from build123d import *

# Parameters (mm, degrees)
BOSS_EXTRUDE1_DEPTH     = 3
FILLET1_R               = 5
CUT_EXTRUDE1_DEPTH      = 165.496200564
CUT_EXTRUDE1_DEPTH_BACK = 165.496200564
SKETCH2_R               = 1.5
CUT_EXTRUDE2_DEPTH      = 165.496200694
CUT_EXTRUDE2_DEPTH_BACK = 165.496200694
SKETCH3_R               = 2.5
CUT_EXTRUDE3_DEPTH      = 165.496200694
CUT_EXTRUDE3_DEPTH_BACK = 165.496200694
SKETCH4_R               = 3.75
SKETCH4_R_2             = 2.75
SKETCH4_W               = 71.5
SKETCH4_H               = 25
SKETCH5_R               = 1.5
BOSS_EXTRUDE2_DEPTH     = 25


with BuildPart() as part:
    # Sketch1 → Boss-Extrude1 (new body)
    with BuildSketch(Plane(origin=(0, 0, 0), x_dir=(1, 0, 0), z_dir=(0, 1, 0))):
        with BuildLine():
            Line((0, 5), (150, 5))
            ThreePointArc((150, 5), (153.535533906, 3.535533906), (155, 0))
            Line((155, 0), (155, -50))
            ThreePointArc((155, -50), (153.535533906, -53.535533906), (150, -55))
            Line((150, -55), (0, -55))
            ThreePointArc((0, -55), (-3.535533906, -53.535533906), (-5, -50))
            Line((-5, -50), (-5, 0))
            ThreePointArc((-5, 0), (-3.535533906, 3.535533906), (0, 5))
        make_face()
    extrude(amount=BOSS_EXTRUDE1_DEPTH)

    # Fillet1
    # the kernel refuses this fillet: 5 mm, written as the material it takes off along each edge
    with BuildSketch(Plane(origin=(0, 3, 50), x_dir=(0, 0, 1), z_dir=(1, 0, 0))) as fillet1_piece_1:
        with BuildLine():
            CenterArc((0.417424305, 5), FILLET1_R, 270, 66.421821522)
            Line((0.417424305, 0), (0.417424305, -0.1))
            Line((0.417424305, -0.1), (5, -0.1))
            Line((5, -0.1), (5.1, 0))
            ThreePointArc((5.1, 0), (5.1, 1.5), (5.091651514, 2.96))
            Line((5.091651514, 2.96), (5, 3))
        make_face()
    revolve(axis=Axis((0, 3, 50), (0, -1, 0)), revolution_arc=90, mode=Mode.SUBTRACT)
    with BuildSketch(Plane(origin=(-5, 3, 50), x_dir=(0, -1, 0), z_dir=(0, 0, -1)), Plane(origin=(155, 3, 0), x_dir=(0, -1, 0), z_dir=(0, 0, 1))) as fillet1_piece_2:
        with BuildLine():
            CenterArc((5, -4.582575695), FILLET1_R, 113.578178478, 66.421821522)
            Line((0, -4.582575695), (-0.1, -4.582575695))
            Line((-0.1, -4.582575695), (-0.1, 0))
            Line((-0.1, 0), (0, 0.1))
            ThreePointArc((0, 0.1), (1.5, 0.1), (2.96, 0.091651514))
            Line((2.96, 0.091651514), (3, 0))
        make_face()
    extrude(amount=50, mode=Mode.SUBTRACT)
    with BuildSketch(Plane(origin=(0, 3, 0), x_dir=(-1, 0, 0), z_dir=(0, 0, 1))) as fillet1_piece_3:
        with BuildLine():
            CenterArc((0.417424305, 5), FILLET1_R, 270, 66.421821522)
            Line((0.417424305, 0), (0.417424305, -0.1))
            Line((0.417424305, -0.1), (5, -0.1))
            Line((5, -0.1), (5.1, 0))
            ThreePointArc((5.1, 0), (5.1, 1.5), (5.091651514, 2.96))
            Line((5.091651514, 2.96), (5, 3))
        make_face()
    revolve(axis=Axis((0, 3, 0), (0, -1, 0)), revolution_arc=90, mode=Mode.SUBTRACT)
    with BuildSketch(Plane(origin=(0, 3, -5), x_dir=(0, -1, 0), z_dir=(1, 0, 0)), Plane(origin=(150, 3, 55), x_dir=(0, -1, 0), z_dir=(-1, 0, 0))) as fillet1_piece_4:
        with BuildLine():
            CenterArc((5, -4.582575695), FILLET1_R, 113.578178478, 66.421821522)
            Line((0, -4.582575695), (-0.1, -4.582575695))
            Line((-0.1, -4.582575695), (-0.1, 0))
            Line((-0.1, 0), (0, 0.1))
            ThreePointArc((0, 0.1), (1.5, 0.1), (2.96, 0.091651514))
            Line((2.96, 0.091651514), (3, 0))
        make_face()
    extrude(amount=150, mode=Mode.SUBTRACT)
    with BuildSketch(Plane(origin=(150, 3, 0), x_dir=(0, 0, -1), z_dir=(-1, 0, 0))) as fillet1_piece_5:
        with BuildLine():
            CenterArc((0.417424305, 5), FILLET1_R, 270, 66.421821522)
            Line((0.417424305, 0), (0.417424305, -0.1))
            Line((0.417424305, -0.1), (5, -0.1))
            Line((5, -0.1), (5.1, 0))
            ThreePointArc((5.1, 0), (5.1, 1.5), (5.091651514, 2.96))
            Line((5.091651514, 2.96), (5, 3))
        make_face()
    revolve(axis=Axis((150, 3, 0), (0, -1, 0)), revolution_arc=90, mode=Mode.SUBTRACT)
    with BuildSketch(Plane(origin=(150, 3, 50), x_dir=(1, 0, 0), z_dir=(0, 0, -1))) as fillet1_piece_6:
        with BuildLine():
            CenterArc((0.417424305, 5), FILLET1_R, 270, 66.421821522)
            Line((0.417424305, 0), (0.417424305, -0.1))
            Line((0.417424305, -0.1), (5, -0.1))
            Line((5, -0.1), (5.1, 0))
            ThreePointArc((5.1, 0), (5.1, 1.5), (5.091651514, 2.96))
            Line((5.091651514, 2.96), (5, 3))
        make_face()
    revolve(axis=Axis((150, 3, 50), (0, -1, 0)), revolution_arc=90, mode=Mode.SUBTRACT)

    # Sketch2 → Cut-Extrude1 (cut, two sides: drawn at the far end of the back side and taken through both)
    with BuildSketch(Plane(origin=(0, 3, 0), x_dir=(1, 0, 0), z_dir=(0, 1, 0)).offset(-CUT_EXTRUDE1_DEPTH_BACK)):
        with Locations(Location((0, -50, 0), (0, 0, 270))):
            Circle(SKETCH2_R)
        with Locations(Location((0, 0, 0), (0, 0, 270))):
            Circle(SKETCH2_R)
        with Locations(Location((150, -50, 0), (0, 0, 270))):
            Circle(SKETCH2_R)
        with Locations(Location((150, 0, 0), (0, 0, 270))):
            Circle(SKETCH2_R)
    extrude(amount=CUT_EXTRUDE1_DEPTH + CUT_EXTRUDE1_DEPTH_BACK, mode=Mode.SUBTRACT)

    # Sketch3 → Cut-Extrude2 (cut, two sides: drawn at the far end of the back side and taken through both)
    with BuildSketch(Plane(origin=(0, 3, 0), x_dir=(1, 0, 0), z_dir=(0, 1, 0)).offset(-CUT_EXTRUDE2_DEPTH_BACK)):
        with Locations(Location((25, -25, 0), (0, 0, 270))):
            Circle(SKETCH3_R)
        with BuildLine():
            ThreePointArc((30.5, -15.473720558), (25, -14), (19.5, -15.473720558))
            ThreePointArc((19.5, -15.473720558), (18.584936491, -18.888784068), (22, -19.803847577))
            ThreePointArc((22, -19.803847577), (25, -19), (28, -19.803847577))
            ThreePointArc((28, -19.803847577), (31.415063509, -18.888784068), (30.5, -15.473720558))
        make_face()
        with BuildLine():
            ThreePointArc((30.5, -34.526279442), (34.526279442, -30.5), (36, -25))
            ThreePointArc((36, -25), (33.5, -22.5), (31, -25))
            ThreePointArc((31, -25), (30.196152423, -28), (28, -30.196152423))
            ThreePointArc((28, -30.196152423), (27.084936491, -33.611215932), (30.5, -34.526279442))
        make_face()
        with BuildLine():
            ThreePointArc((14, -25), (15.473720558, -30.5), (19.5, -34.526279442))
            ThreePointArc((19.5, -34.526279442), (22.915063509, -33.611215932), (22, -30.196152423))
            ThreePointArc((22, -30.196152423), (19.803847577, -28), (19, -25))
            ThreePointArc((19, -25), (16.5, -22.5), (14, -25))
        make_face()
        with BuildLine():
            ThreePointArc((34.75, -8.112504626), (25, -5.5), (15.25, -8.112504626))
            ThreePointArc((15.25, -8.112504626), (14.334936491, -11.527568136), (17.75, -12.442631645))
            ThreePointArc((17.75, -12.442631645), (25, -10.5), (32.25, -12.442631645))
            ThreePointArc((32.25, -12.442631645), (35.665063509, -11.527568136), (34.75, -8.112504626))
        make_face()
        with BuildLine():
            ThreePointArc((34.75, -41.887495374), (41.887495374, -34.75), (44.5, -25))
            ThreePointArc((44.5, -25), (42, -22.5), (39.5, -25))
            ThreePointArc((39.5, -25), (37.557368355, -32.25), (32.25, -37.557368355))
            ThreePointArc((32.25, -37.557368355), (31.334936491, -40.972431864), (34.75, -41.887495374))
        make_face()
        with BuildLine():
            ThreePointArc((5.5, -25), (8.112504626, -34.75), (15.25, -41.887495374))
            ThreePointArc((15.25, -41.887495374), (18.665063509, -40.972431864), (17.75, -37.557368355))
            ThreePointArc((17.75, -37.557368355), (12.442631645, -32.25), (10.5, -25))
            ThreePointArc((10.5, -25), (8, -22.5), (5.5, -25))
        make_face()
    extrude(amount=CUT_EXTRUDE2_DEPTH + CUT_EXTRUDE2_DEPTH_BACK, mode=Mode.SUBTRACT)

    # Sketch4 → Cut-Extrude3 (cut, two sides: drawn at the far end of the back side and taken through both)
    with BuildSketch(Plane(origin=(0, 3, 0), x_dir=(1, 0, 0), z_dir=(0, 1, 0)).offset(-CUT_EXTRUDE3_DEPTH_BACK)):
        with Locations(Location((59.917424305, -35.417424305, 0), (0, 0, 270))):
            Circle(SKETCH4_R)
        with Locations(Location((59.917424305, -9.417424305, 0), (0, 0, 270))):
            Circle(SKETCH4_R_2)
        with Locations((110.667424305, -27.917424305)):
            Rectangle(SKETCH4_W, SKETCH4_H)
    extrude(amount=CUT_EXTRUDE3_DEPTH + CUT_EXTRUDE3_DEPTH_BACK, mode=Mode.SUBTRACT)

    # Sketch5 → Boss-Extrude2 (add)
    with BuildSketch(Plane.XZ):
        with BuildLine():
            Line((155, 0), (155, 50))
            ThreePointArc((155, 50), (153.535533906, 53.535533906), (150, 55))
            Line((150, 55), (0, 55))
            ThreePointArc((0, 55), (-3.535533906, 53.535533906), (-5, 50))
            Line((-5, 50), (-5, 0))
            ThreePointArc((-5, 0), (-3.535533906, -3.535533906), (0, -5))
            Line((0, -5), (150, -5))
            ThreePointArc((150, -5), (153.535533906, -3.535533906), (155, 0))
        make_face()
        with Locations(Location((0, 50, 0), (0, 0, 90))):
            Circle(SKETCH5_R, mode=Mode.SUBTRACT)
        with Locations(Location((0, 0, 0), (0, 0, 270))):
            Circle(SKETCH5_R, mode=Mode.SUBTRACT)
        with Locations(Location((150, 0, 0), (0, 0, 270))):
            Circle(SKETCH5_R, mode=Mode.SUBTRACT)
        with Locations(Location((150, 50, 0), (0, 0, 90))):
            Circle(SKETCH5_R, mode=Mode.SUBTRACT)
        with BuildLine():
            Line((4, 53), (146, 53))
            ThreePointArc((146, 53), (146.464466094, 46.464466094), (153, 46))
            Line((153, 46), (153, 4))
            ThreePointArc((153, 4), (146.464466094, 3.535533906), (146, -3))
            Line((146, -3), (4, -3))
            ThreePointArc((4, -3), (3.535533906, 3.535533906), (-3, 4))
            Line((-3, 4), (-3, 46))
            ThreePointArc((-3, 46), (3.535533906, 46.464466094), (4, 53))
        make_face(mode=Mode.SUBTRACT)
    extrude(amount=BOSS_EXTRUDE2_DEPTH)


solid = part.part
Build history of the part. All positions in model axes, mm. A direction names the side the tool comes from. Coordinates: 2 decimals unless noted, no trailing zeros. Order: outer loops, then holes, each group sorted by start corner. A loop starts at its lowest first (then second) coordinate and runs counter-clockwise, first axis right, second up. Notation, with made-up numbers: (40.5, -39.75) - (56.5, -39.75) arc R26 ccw to (56.5, -17.75) - close; hole circle Ø3 at (-14.5, 77). An arc over 180 degrees is marked (long way). Write each question's results on one line, items separated by ' | '. Start each with the question number.
Item 1: Flat gauge pins, fed straight in: pin 1 (1.5 mm diameter, centred on x = 118, y = 1, fed in from -Z); pin 2 (1.5 mm diameter, centred on y = 1.5, z = 28, fed in from -X); pin 3 (2.5 mm diameter, centred on x = 150, z = 50, fed in from -Y); pin 4 (3 mm diameter, centred on x = 78, z = 49, fed in from -Y). Where does each tip first touch, or does it go through?
Item 2: Band-saw the part on C-C on x = 42. Write the cut outline in (y, z), and give its area (3 significant figures).
Item 3: Band-saw the part on A-A on x = 91. Write the cut outline in (y, z).
Item 4: Wall check: probe 1 along X at (y, z) = (-6.25, 0); probe 2 along X at (y, z) = (-23, 8); probe 3 along Z at (x, y) = (54, -9). Give the ranges that are in metal, low to high. Write a range as [from, to].
Item 5: Band-saw the part on B-B on y = -13.5. Write the cut outline in (x, z), and give its area (3 significant figures).
Item 6: Mould opens along Z. For faces 4 (the face through (75, -25, -4)), 5 (the face through (73.95, 2.16, -3.19)), 6 (the face through (146, -12, 47)) say: released by +Z, released by -Z, zero draft, split by the parting line, or undercut.
Item 7: Tool access for faces 1 (the face through (155, -12, 25)), 2 (the face through (25, 1, 14)), 3 (the face through (59, 0, 25)): list every direction of +Z, -Z, +X, -X, +Y, -Y with a clear straight run to the whole face (end or side of a thin tool).
Numbers:
1) pin 1: z = -4.88 | pin 2: x = -4.59 | pin 3: through | pin 4: y = 0
2) outline: (-25, -5) - (0, -5) arc R5 ccw to (3, -0.42) - (3, 22.5) - (0, 22.5) - (0, -3) - (-25, -3) - close; (-25, 53) - (0, 53) - (0, 34.55) - (3, 34.55) - (3, 50.42) arc R5 ccw to (0, 55) - (-25, 55) - close | area: 236 mm^2
3) outline: (-25, -5) - (0, -5) arc R5 ccw to (3, -0.42) - (3, 15.42) - (0, 15.42) - (0, -3) - (-25, -3) - close; (-25, 53) - (0, 53) - (0, 40.42) - (3, 40.42) - (3, 50.42) arc R5 ccw to (0, 55) - (-25, 55) - close
4) probe 1: [-5, -1.5], [1.5, 5], [145, 148.5], [151.5, 155] | probe 2: [-5, -3], [153, 155] | probe 3: [-5, -3], [53, 55]
5) outline: (-5, 0) arc R5 ccw to (0, -5) - (150, -5) arc R5 ccw to (155, 0) - (155, 50) arc R5 ccw to (150, 55) - (0, 55) arc R5 ccw to (-5, 50) - close; hole (-3, 4) arc R5 cw to (4, -3) - (146, -3) arc R5 cw to (153, 4) - (153, 46) arc R5 cw to (146, 53) - (4, 53) arc R5 cw to (-3, 46) - close; hole circle Ø3 at (0, 0); hole circle Ø3 at (0, 50); hole circle Ø3 at (150, 0); hole circle Ø3 at (150, 50) | area: 1,040 mm^2
6) face 4: zero draft | face 5: released by -Z | face 6: undercut
7) face 1: +Z, -Z, +X, +Y, -Y | face 2: +Y, -Y | face 3: -Y
